Part model, mm, in its own coordinate system. Round coordinates to 2 decimals unless told otherwise and drop trailing zeros. Write each loop counter-clockwise with the first axis right and the second up, starting at its lowest first coordinate (ties: lowest second). Pieces come first, ordered by that corner, then holes. Notation, with made-up numbers: M -36.5,25.5 L 5.5,25.5 A23 ccw 5.5,38.5 Z; hole C 46.25,9.25 d9. An arc over 180 degrees is marked long. Use a Markdown table: item, result. Add a question column.
1) Two-plate mould, pull along X, no slides. Class faces 1 (the face through (-4.143, 1.801, 0.315)), 2 (the face through (0, -2, 2)), 3 (the face through (-0.1, 2.3, 5)): released by +X, released by -X, zero draft, split by the parting line, or undercut.
2) Slice it at C-C on x = 0. Write the cut outline in (y, z), plus the area to 3 significant figures.
3) Slice it at B-B on y = 0. Write the cut outline in (x, z).
4) Drop flat-ended pins along their axis: P1, Ø1, axis at x = 2.5, z = 1, coming from the +Y side; P2, Ø1, axis at x = 2.5, z = 2, coming from the -Y side; P3, Ø1.5, axis at x = -2, z = 4, coming from the -Y side; P4, Ø2.5, axis at x = 0, y = 0, coming from the +Z side. Give the stop position or say it passes through.
5) Slice it at A-A on z = 3.3. Write the cut outline in (x, y), plus the area to 3 significant figures.
6) Wall check: probe 1 along Y at (x, z) = (0, 2.3); probe 2 along Y at (x, z) = (1.5, 2.05); probe 3 along X at (y, z) = (-0.5, 2.7). Give the ranges that are in metal, low to high.
```python
from build123d import *

# Parameters (mm, degrees)
BOSS_EXTRUDE2_DEPTH = 5
SKETCH2_R           = 2
CUT_EXTRUDE1_DEPTH  = 9.440506234
SKETCH3_OUTSIDE_W   = 19.212
SKETCH3_OUTSIDE_H   = 19.994
SKETCH3_OUTSIDE_R   = 4.356968777
CUT_EXTRUDE2_DEPTH  = 5
CUT_EXTRUDE2_DRAFT  = -27


with BuildPart() as part:
    # Sketch1 → Boss-Extrude2 (new body)
    with BuildSketch(Plane.XY):
        Polygon((4.608920208, -2.017116032), (4.05133383, 2.982883968), (-0.557586378, 5), (-4.608920208, 2.017116032), (-4.05133383, -2.982883968), (0.557586378, -5), align=None)
    extrude(amount=BOSS_EXTRUDE2_DEPTH)

    # Sketch2 → Cut-Extrude1 (cut, through all)
    with BuildSketch(Plane(origin=(0, 0, 0), x_dir=(-1, 0, 0), z_dir=(0, 0, -1))):
        Circle(SKETCH2_R)
    extrude(amount=-CUT_EXTRUDE1_DEPTH, mode=Mode.SUBTRACT)


with BuildPart() as cut_extrude2_tool:
    # Sketch3 outside → Cut-Extrude2 (with draft: the straight prism first)
    with BuildSketch(Plane(origin=(0, 0, 0), x_dir=(-1, 0, 0), z_dir=(0, 0, -1))):
        Rectangle(SKETCH3_OUTSIDE_W, SKETCH3_OUTSIDE_H)
        Circle(SKETCH3_OUTSIDE_R, mode=Mode.SUBTRACT)
    extrude(amount=-CUT_EXTRUDE2_DEPTH)
    # Cut-Extrude2: the draft: its side faces are tilted about the plane it starts from
    cut_extrude2_sides = [cut_extrude2_tool.faces().sort_by_distance(p)[0] for p in [
        (0, -9.997, 2.5),
        (-9.606, 0, 2.5),
        (0, 9.997, 2.5),
        (9.606, 0, 2.5),
        (4.356968777, 0, 2.5),
    ]]
    draft(cut_extrude2_sides, Plane(origin=(0, 0, 0), x_dir=(-1, 0, 0), z_dir=(0, 0, -1)), CUT_EXTRUDE2_DRAFT)


with BuildPart() as part_1:
    add(part.part)

    # Cut-Extrude2: cut by cut_extrude2_tool
    add(cut_extrude2_tool.part, mode=Mode.SUBTRACT)


solid = part_1.part
```
Entries:
| question | item | result |
|---|---|---|
| 1 | face 1 | released by -X |
| 1 | face 2 | undercut |
| 1 | face 3 | zero draft |
| 2 | outline | M -4.76,0.78 L -4.36,0 L -2,0 L -2,5 L -4.76,5 Z; M 2,0 L 4.36,0 L 4.76,0.78 L 4.76,5 L 2,5 Z |
| 2 | area | 27.2 mm^2 |
| 3 | outline | M -4.38,0.05 L -4.36,0 L -2,0 L -2,5 L -4.38,5 Z; M 2,0 L 4.36,0 L 4.38,0.05 L 4.38,5 L 2,5 Z |
| 4 | P1 | stops at y = 3.88 |
| 4 | P2 | stops at y = -3.94 |
| 4 | P3 | stops at y = -4.21 |
| 4 | P4 | passes through |
| 5 | outline | M -4.61,2.02 L -4.05,-2.98 L 0.56,-5 L 4.61,-2.02 L 4.05,2.98 L -0.56,5 Z; hole C 0,0 d4 |
| 5 | area | 53.2 mm^2 |
| 6 | probe 1 | y = -4.76 to -2, 2 to 4.76 |
| 6 | probe 2 | y = -4.31 to -1.32, 1.32 to 4.1 |
| 6 | probe 3 | x = -4.33 to -1.94, 1.94 to 4.44 |
